Geometry check sheet. Reference: the model listing, model coordinates, mm. Round coordinates to 2 decimals unless told otherwise and drop trailing zeros. Order: outer loops, then holes, each group sorted by start corner. A loop starts at its lowest first (then second) coordinate and runs counter-clockwise, first axis right, second up. Notation, with made-up numbers: (77.25, -39.5) - (126.25, -39.5) arc R14 ccw to (126.25, -21.5) - close; hole circle Ø1 at (28, -16). An arc over 180 degrees is marked (long way). Use a Markdown table: item, result. Add a question column.
(1) Section check A-A on z = -12.7. Record the boundary of the cut face in (x, y) (3 decimals), then the cut area to 3 significant figures.
(2) Thickness scan on line 1 along Y through (x, z) = (6, -512.5) (3 decimals); line 2 along Y through (x, z) = (0.85, -552.45); line 3 along X through (y, z) = (30, -520). Record the ranges inside material, lowest first. Write a range as [from, to].
(3) Gauge pin test, flat ends, axial feed: P1, Ø5, axis at y = 22, z = -73.5, coming from the +X side; P2, Ø2, axis at y = 27, z = -307.5, coming from the +X side. Record the tip position at first contact, or that the pin passes through.
Autodesk Inventor part; units mm, degrees
ref_plane "YZ Plane" through (0, 0, 0) normal (1, 0, 0) x (0, 1, 0)
ref_plane "XZ Plane" through (0, 0, 0) normal (0, 1, 0) x (-1, 0, 0)
ref_plane "XY Plane" through (0, 0, 0) normal (0, 0, 1) x (1, 0, 0)
sketch "Sketch1" plane through (0, 0, 0) normal (0, 0, 1) x (1, 0, 0)
  line L0 (5.9771, 0) -> (28.2021, 0)
  line L1 (28.2021, 0) -> (28.2021, 3.175)
  line L2 (28.2021, 3.175) -> (5.9771, 3.175)
  line L3 (2.8021, 6.35) -> (2.8021, 25.4)
  line L4 (5.9771, 28.575) -> (28.2021, 28.575)
  line L5 (28.2021, 28.575) -> (28.2021, 31.75)
  line L6 (28.2021, 31.75) -> (5.9771, 31.75)
  line L7 (-0.3729, 25.4) -> (-0.3729, 6.35)
  arc A0 (5.9771, 28.575) -> (2.8021, 25.4) centre (5.9771, 25.4) ccw
  arc A1 (2.8021, 6.35) -> (5.9771, 3.175) centre (5.9771, 6.35) ccw
  arc A2 (5.9771, 31.75) -> (-0.3729, 25.4) centre (5.9771, 25.4) ccw
  arc A3 (-0.3729, 6.35) -> (5.9771, 0) centre (5.9771, 6.35) ccw
  point P0 (0, 0)
  point P1 (-0.3729, 0)
  point P2 (2.8021, 3.175)
  point P3 (2.8021, 28.575)
  dimension "d0" = 28.575
  dimension "d1" = 3.175
  dimension "d2" = 25.4
  dimension "d3" = 25.4
  dimension "d4" = 3.175
  dimension "d5" = 3.175
  dimension "d6" = 6.35
extrude "Extrusion1" add sketch "Sketch1" against normal blind 609.6
sketch "Sketch2" plane through (-0.3729, 6.35, 0) normal (-1, 0, 0) x (0, 0, 1)
  line L0 (0, 19.05) -> (-609.6, 19.05)
  line L1 (-228.6, 0) -> (-228.6, 7.9375)
  arc A0 (-228.6, 11.1125) -> (-228.6, 7.9375) centre (-228.6, 9.525) ccw
  line L2 (-228.6, 11.1125) -> (-228.6, 19.05)
  line L3 (-228.6, 19.05) -> (-889, 19.05)
  line L4 (-889, 0) -> (-889, 19.05)
  line L5 (-889, 0) -> (-228.6, 0)
  circle A1 centre (-552.45, 11.43) radius 4.826
  circle A2 centre (-501.65, 11.43) radius 4.826
  circle A3 centre (-387.35, 11.43) radius 4.826
  circle A4 centre (-336.55, 11.43) radius 4.826
  circle A5 centre (-444.5, 7.62) radius 4.826
  circle A6 centre (-730.25, 11.43) radius 4.826
  circle A7 centre (-781.05, 11.43) radius 4.826
  line L6 (0, 25.4) -> (-609.6, 25.4) construction
  circle A8 centre (-133.35, 11.43) radius 4.826
  circle A9 centre (-82.55, 11.43) radius 4.826
  point P0 (0, -6.35)
  point P1 (-254, 0.852)
  dimension "d10" = 7.62
  dimension "d11" = 3.81
  dimension "d14" = 254
hole "Hole1" at (-0.3729, 17.78, -781.05) at (-0.3729, 17.78, -730.25) at (-0.3729, 17.78, -552.45) at (-0.3729, 17.78, -501.65) at (-0.3729, 13.97, -444.5) at (-0.3729, 17.78, -387.35) at (-0.3729, 17.78, -336.55) at (-0.3729, 17.78, -133.35) at (-0.3729, 17.78, -82.55) direction (1, 0, 0) diameter 9.652 end through all
hole "Hole2" at (-0.3729, 15.875, -228.6) direction (1, 0, 0) diameter 3.175 end through all
sketch "Sketch3" plane through (5.9771, 31.75, 0) normal (0, 1, 0) x (1, 0, 0)
  line L0 (22.225, 609.6) -> (0, 609.6)
  line L1 (22.225, 0) -> (22.225, 609.6)
  point P0 (-5.9771, 0)
  point P1 (9.525, 596.9)
  dimension "d34" = 12.7
  dimension "d35" = 12.7
hole "Hole3" at (15.5021, 31.75, -596.9) direction (0, -1, 0) diameter 6.5278 end through all
pattern_linear "Rectangular Pattern1" count 35 spacing 25.4 along (0, 0, 1) of "Hole3"
hole "Hole4" at (15.5021, 31.75, -12.7) direction (0, -1, 0) diameter 12.7 end through all
hole "Hole5" at (15.5021, 31.75, -596.9) direction (0, -1, 0) diameter 12.7 end through all
properties part number "c-channel (24 in with .5 in holes)"
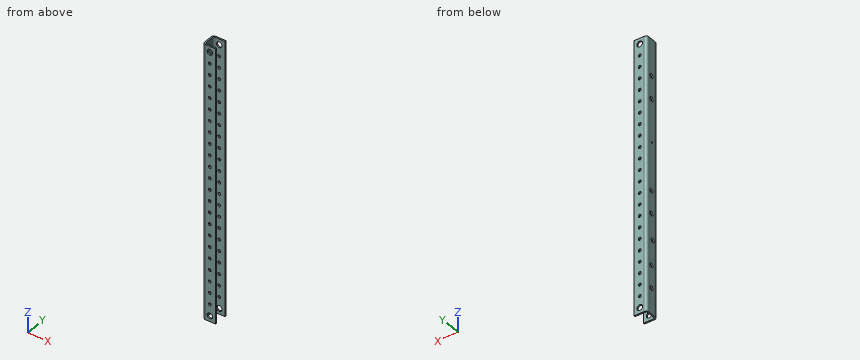
Check sheet entries:
| question | item | result |
|---|---|---|
| 1 | outline | (-0.373, 6.35) arc R6.35 ccw to (5.977, 0) - (9.152, 0) - (9.152, 3.175) - (5.977, 3.175) arc R3.175 cw to (2.802, 6.35) - (2.802, 25.4) arc R3.175 cw to (5.977, 28.575) - (9.152, 28.575) - (9.152, 31.75) - (5.977, 31.75) arc R6.35 ccw to (-0.373, 25.4) - close; (21.852, 0) - (28.202, 0) - (28.202, 3.175) - (21.852, 3.175) - close; (21.852, 28.575) - (28.202, 28.575) - (28.202, 31.75) - (21.852, 31.75) - close |
| 1 | area | 168 mm2 |
| 2 | line 1 | y = [0, 3.175], [28.575, 31.75] |
| 2 | line 2 | y = [2.6, 12.95], [22.61, 29.15] |
| 2 | line 3 | x = [1.6, 12.31], [18.69, 28.2] |
| 3 | P1 | stops at x = 2.8 |
| 3 | P2 | stops at x = 4.15 |
